Here's how the part is built. I have some questions about the finished solid (model axes, mm). A direction names the side the tool comes from. Round coordinates to 2 decimals unless told otherwise and drop trailing zeros. Order: outer loops, then holes, each group sorted by start corner. A loop starts at its lowest first (then second) coordinate and runs counter-clockwise, first axis right, second up. Notation, with made-up numbers: (-10.5, 83) - (44.5, 83) arc R10 cw to (44.5, 100) - close; hole circle Ø7 at (-20, 33). An arc over 180 degrees is marked (long way). One line per item, written item: value.
Autodesk Inventor part; units mm, degrees
ref_plane "YZ Plane" through (0, 0, 0) normal (1, 0, 0) x (0, 1, 0)
ref_plane "XZ Plane" through (0, 0, 0) normal (0, 1, 0) x (-1, 0, 0)
ref_plane "XY Plane" through (0, 0, 0) normal (0, 0, 1) x (1, 0, 0)
sketch "Sketch1" plane through (0, 0, 0) normal (0, 1, 0) x (-1, 0, 0)
  line L0 (0, 0) -> (65, 0)
  line L1 (65, 0) -> (65, -200)
  line L2 (65, -200) -> (0, -200)
  line L3 (0, -200) -> (0, 0)
  dimension "d0" = 65
  dimension "d1" = 200
extrude "Extrusion1" add sketch "Sketch1" along normal blind 18
sketch "Sketch2" plane through (0, 18, 0) normal (0, 1, 0) x (1, 0, 0)
  line L0 (0, 0) -> (0, 200)
  line L1 (0, 0) -> (-32.5, 0)
  line L2 (-65, 0) -> (0, 0)
  line L3 (-32.5, 0) -> (-32.5, 8)
  line L4 (-32.5, 8) -> (-55.5, 8)
  line L5 (-55.5, 8) -> (-55.5, 18.5)
  line L6 (-55.5, 18.5) -> (-9.5, 18.5)
  line L7 (-9.5, 18.5) -> (-9.5, 8)
  line L8 (-9.5, 8) -> (-32.5, 8)
  dimension "d4" = 8
  dimension "d5" = 23
  dimension "d6" = 10.5
  dimension "d7" = 46
  dimension "d8" = 10.5
extrude "Extrusion2" cut sketch "Sketch2" against normal through all
sketch "Sketch3" plane through (0, 18, 0) normal (0, 1, 0) x (1, 0, 0)
  line L0 (-55.5, 18.5) -> (-9.5, 18.5)
  line L1 (-32.5, 18.5) -> (-32.5, 135)
  circle A0 centre (-32.5, 135) radius 23.75
  point P0 (0, 0)
  dimension "d11" = 116.5
  dimension "d12" = 47.5
extrude "Extrusion3" cut sketch "Sketch3" against normal blind 12.5
sketch "Sketch4" plane through (-32.5, 5.5, -135) normal (0, 1, 0) x (1, 0, 0)
  circle A0 centre (0, 0) radius 14
  point P0 (32.5, -135)
  dimension "d15" = 28
extrude "Extrusion4" cut sketch "Sketch4" against normal blind 4
sketch "Sketch7" plane through (0, 18, 0) normal (0, 1, 0) x (1, 0, 0)
  line L0 (0, 200) -> (-65, 200)
  line L1 (-65, 200) -> (0, 200)
  line L2 (-32.5, 200) -> (-32.5, 158.75)
  circle A0 centre (-32.5, 135) radius 23.75
  line L3 (-32.5, 200) -> (-11, 200)
  line L4 (-11, 200) -> (-54, 200)
  line L5 (0, 0) -> (0, 200)
  line L6 (-11, 200) -> (-11, 158.75)
  line L7 (-54, 200) -> (-54, 158.75)
  line L8 (-54, 158.75) -> (-65, 158.75)
  line L9 (-65, 200) -> (-65, 0)
  line L10 (-65, 200) -> (-54, 200)
  line L11 (-11, 158.75) -> (0, 158.75)
  line L12 (0, 200) -> (0, 158.75)
  line L13 (0, 200) -> (-11, 200)
  dimension "d19" = 21.5
  dimension "d20" = 43
extrude "Extrusion5" add sketch "Sketch7" along normal blind 39.5 contours L5 L11 L6 L0 | L7 L8 L9 L0
sketch "Sketch8" plane through (0, 57.5, 0) normal (0, 1, 0) x (1, 0, 0)
  line L0 (0, 0) -> (0, 200)
  line L1 (-11, 200) -> (-54, 200)
  line L2 (0, 200) -> (-11, 200)
  line L3 (0, 200) -> (-65, 200)
  line L4 (-11, 200) -> (-20, 200)
  line L5 (-20, 200) -> (-20, 158.75)
  line L6 (-20, 158.75) -> (0, 158.75)
  line L7 (0, 200) -> (0, 158.75)
  line L8 (-65, 158.75) -> (-54.25, 158.75)
  line L9 (-54.25, 158.75) -> (-45.25, 158.75)
  line L10 (-45.25, 158.75) -> (-45.25, 200)
  line L11 (-54, 200) -> (-65, 200)
  line L12 (-65, 200) -> (-45.25, 200)
  line L13 (-65, 159.6209) -> (-65, 200)
  line L14 (-65, 200) -> (-65, 158.75)
  line L15 (-65, 200) -> (-65, 158.75)
  dimension "d23" = 9
  dimension "d24" = 9
extrude "Extrusion6" add sketch "Sketch8" along normal blind 10
sketch "Sketch10" plane through (0, 0, -200) normal (0, 0, -1) x (-1, 0, 0)
  line L0 (20, 57.5) -> (11, 57.5)
  line L1 (20, 57.5) -> (20, 67.5)
  line L2 (20, 57.5) -> (20, 67.5)
  line L3 (20, 67.5) -> (0, 67.5)
  line L4 (20, 67.5) -> (0, 67.5)
  line L5 (0, 67.5) -> (0, 0)
  line L6 (0, 0) -> (65, 0)
  line L7 (0, 0) -> (65, 0)
  line L8 (65, 0) -> (65, 67.5)
  line L9 (65, 0) -> (65, 67.5)
  line L10 (45.25, 67.5) -> (65, 67.5)
  line L11 (65, 67.5) -> (45.25, 67.5)
  line L12 (45.25, 57.5) -> (45.25, 67.5)
  line L13 (45.25, 67.5) -> (45.25, 57.5)
  line L14 (45.25, 57.5) -> (54, 57.5)
  line L15 (45.25, 57.5) -> (54, 57.5)
  line L16 (54, 18) -> (54, 57.5)
  line L17 (54, 57.5) -> (54, 18)
  line L18 (11, 18) -> (11, 57.5)
  line L19 (54, 18) -> (11, 18)
  line L20 (11, 18) -> (11, 57.5)
  line L21 (11, 57.5) -> (20, 57.5)
extrude "Extrusion7" add sketch "Sketch10" along normal blind 40
sketch "Sketch14" plane through (0, 0, 0) normal (1, 0, 0) x (0, 0, -1)
  line L0 (240, 67.5) -> (240, 57.5)
  line L1 (240, 67.5) -> (228.3141, 67.5)
  line L2 (158.75, 67.5) -> (240, 67.5)
  line L3 (228.3141, 67.5) -> (228.3141, 18)
  line L4 (240, 18) -> (158.75, 18)
  line L5 (228.3141, 18) -> (218.3141, 18)
  line L6 (218.3141, 18) -> (218.3141, 67.5)
  line L7 (218.3141, 67.5) -> (228.3141, 67.5)
  line L8 (218.3141, 67.5) -> (218.3141, 57.5)
  line L9 (218.3141, 57.5) -> (228.3141, 57.5)
  line L10 (158.75, 57.5) -> (240, 57.5)
  point P0 (0, 0)
  dimension "d29" = 10
extrude "Extrusion8" cut sketch "Sketch14" against normal through all contours L3 L4 L6 L9
sketch "Sketch17" plane through (0, 18, 0) normal (0, 1, 0) x (1, 0, 0)
  line L0 (0, 158.75) -> (0, 240)
  line L1 (0, 240) -> (0, 110)
  line L2 (0, 0) -> (0, 240)
  line L3 (0, 110) -> (0, 90)
  line L4 (0, 90) -> (-15, 90)
  line L5 (-65, 0) -> (-65, 240)
  line L6 (-15, 90) -> (-15, 110)
  line L7 (-15, 110) -> (0, 110)
  line L8 (-15, 90) -> (-15, 80)
  line L9 (-65, 80) -> (-65, 110)
  line L10 (-65, 110) -> (-50, 110)
  line L11 (-50, 110) -> (-50, 80)
  line L12 (-50, 80) -> (-15, 80)
  line L13 (-65, 80) -> (-65, 0)
  line L14 (-65, 0) -> (0, 0)
  line L15 (0, 0) -> (0, 110)
  dimension "d33" = 130
  dimension "d34" = 20
  dimension "d35" = 15
  dimension "d36" = 10
  dimension "d37" = 15
  dimension "d38" = 30
extrude "Extrusion9" cut sketch "Sketch17" against normal through all
sketch "Sketch18" plane through (-50, 18, -80) normal (0, 0, 1) x (1, 0, 0)
  point P0 (50, -18)
sketch "Sketch19" plane through (0, 18, 0) normal (0, 1, 0) x (1, 0, 0)
  point P0 (0, 0)
sketch "Sketch20" plane through (-50, 18, -110) normal (-1, 0, 0) x (0, 0, 1)
  point P0 (110, -18)
sketch "Sketch21" plane through (0, 18, 0) normal (0, 1, 0) x (1, 0, 0)
  point P0 (0, 0)
ref_plane "Work Plane1" through (-32.5, 18, -158.75) normal (-1, 0, 0) x (0, 0, 1)
ref_plane "Work Plane2" through (-32.5, 18, -158.75) normal (1, 0, 0) x (0, 0, -1)
equation "\"BendRadius\" = Thickness"
equation "\"BendReliefWidth\" = Thickness"
equation "\"BendReliefDepth\" = 0.5 * Thickness"
equation "\"CornerReliefSize\" = 4 * Thickness"
equation "\"MinimumRemnant\" = 2 * Thickness"
equation "\"TransitionRadius\" = BendRadius"
equation "\"JacobiRadiusSize\" = BendRadius"
equation "\"GapSize\" = Thickness"
properties part number "techo"
Q1. If we section it at D-D, the plane y = 31.5: Please give me the cut outline in (x, z).
Results list:
outline: (-65, -240) - (-54, -240) - (-54, -228.31) - (-65, -228.31) - close; (-65, -218.31) - (-54, -218.31) - (-54, -158.75) - (-65, -158.75) - close; (-11, -240) - (0, -240) - (0, -228.31) - (-11, -228.31) - close; (-11, -218.31) - (0, -218.31) - (0, -158.75) - (-11, -158.75) - close
Q2. Will these pins go through, and if not, where does the flat tip stop? pin 1 (3.5 mm diameter, centred on x = -7, y = 32, fed in from +Z); pin 2 (12 mm diameter, centred on x = -8, y = 11, fed in from +Z); pin 3 (8 mm diameter, centred on x = -34.5, z = -213.5, fed in from +Y); pin 4 (5 mm diameter, centred on x = -42, y = 21, fed in from -Z).
Results list:
pin 1: z = -158.75
pin 2: z = -110
pin 3: y = 18
pin 4: through
Q3. We'd pull the mould along Y, two halves only. Please class faces 5 (the flat face through (-59, 38, -228.314)), 6 (the flat face through (-32, 0, -159)), 7 (the flat face through (-33, 9, -80)), 8 (the flat face through (-55, 67.5, -199)): released by +Y, released by -Y, zero draft, split by the parting line, or undercut.
Results list:
face 5: undercut
face 6: released by -Y
face 7: zero draft
face 8: released by +Y
Q4. If I drill on line 1 along X through (y, z) = (4.65, -135); line 2 along Z through (x, y) = (-32.5, 12); line 3 along Y through (x, z) = (-50.5, -206.5), over which ranges is the centre line in solid material (lowest first)?
Results list:
line 1: -65 to -46.5, -18.5 to 0
line 2: -240 to -158.75, -111.25 to -80
line 3: 0 to 18, 57.5 to 67.5
Q5. If we section it at A-A, the plane y = 14.5: Please give me the cut outline in (x, z).
Results list:
outline: (-65, -240) - (0, -240) - (0, -110) - (-15, -110) - (-15, -80) - (-50, -80) - (-50, -110) - (-65, -110) - close; hole circle Ø47.5 at (-32.5, -135)
Q6. Which directions (+Z, -Z, +X, -X, +Y, -Y) give clear straight access to the entire face, cutting with the end or side of a thin tool? Please do faces 1 (the flat face through (-20, 62, -199)), 2 (the cylindrical face through (-34.32, 3.53, -148.88)), 3 (the flat face through (-58, 9, -110)), 4 (the flat face through (-54, 37, -188)).
Results list:
face 1: +Z, -Z, +Y
face 2: +Y
face 3: +Z, -X, +Y, -Y
face 4: +Z, -Z
Q7. If we section it at C-C, the plane x = -6.5: Please give me the cut outline in (y, z).
Results list:
outline: (0, -240) - (67.5, -240) - (67.5, -158.75) - (18, -158.75) - (18, -110) - (0, -110) - close; hole (18, -228.31) - (57.5, -228.31) - (57.5, -218.31) - (18, -218.31) - close
Q8. If we section it at B-B, the plane y = 59.5: Please give me the cut outline in (x, z).
Results list:
outline: (-65, -240) - (-45.25, -240) - (-45.25, -158.75) - (-65, -158.75) - close; (-20, -240) - (0, -240) - (0, -158.75) - (-20, -158.75) - close
